Can you work these out from the model? Positions are in its coordinate system, mm. A direction names the side the tool comes from. Give positions to 0.01 mm unless a question says otherwise; leave off trailing zeros. Loops run counter-clockwise (first coordinate to the right, second up) from the corner with the lowest first, then second, coordinate; pieces in that order, holes last. Notation, with made-up numbers: M -12,43 L 8,43 A29 ccw 8,67 Z; hole C 85,-28 d10. An arc over 180 degrees is marked long. Put each result on its own line as item: value. Start each with the question number.
1) Imagine slicing it at D-D (z = 18). Write out the boundary of the cut face in (x, y), then the cut area to 3 significant figures.
2) If we mould it in two halves opening along Y, with no side actions, what happens to faces 1 (the flat face through (-24, -25, 12)), 2 (the flat face through (0, 3, 9)), 3 (the flat face through (0, 6, 0))? For each: +Y half, -Y half, draft (parallel to the pull), parting line (faces both ways), or undercut.
3) For P1, Ø10, axis at y = -48, z = -5, coming from the +X side; P2, Ø20, axis at x = 5, z = -0.5, coming from the -Y side; P3, Ø3, axis at x = 14.5, y = 4, coming from the +Z side; P4, Ø1.5, axis at x = -25.5, y = -4, coming from the -Z side, each with a flat end and sliding along its axis, tell me the tip position at first contact or that it passes through.
4) Imagine slicing it at C-C (x = 13). Write out the boundary of the cut face in (y, z).
5) For faces 4 (the flat face through (-27, -37, -4)), 5 (the cylindrical face through (-29.458, -20.062, 26.795)), 6 (the flat face through (-20.5, -40, 12)), which set-ups out of +Z, -Z, +X, -X, +Y, -Y let a thin tool reach every point of the face, with its end or its side?
6) Imagine slicing it at B-B (y = -32.5). Write out the boundary of the cut face in (x, z).
7) Please list where these lines run through material, in increasing order: line 1 along X through (y, z) = (-9, 2.5); line 2 along X through (y, z) = (-43.5, 20); line 3 along Y through (x, z) = (18, -6). Write a range as from..to.
8) Imagine slicing it at A-A (z = 6.5). Write out the boundary of the cut face in (x, y), then the cut area to 3 significant figures.
from build123d import *

# Parameters (mm, degrees)
SKETCH1_W           = 65
SKETCH1_H           = 18
BOSS_EXTRUDE1_DEPTH = 6
BOSS_EXTRUDE2_DEPTH = 6
FILLET1_R           = 10
FILLET3_R           = 3
SKETCH3_W           = 31
SKETCH3_H           = 31
BOSS_EXTRUDE3_DEPTH = 6


with BuildPart() as part:
    # Sketch1 → Boss-Extrude1 (new body)
    with BuildSketch(Plane(origin=(0, 0, 0), x_dir=(1, 0, 0), z_dir=(0, 1, 0))):
        Rectangle(SKETCH1_W, SKETCH1_H)
    extrude(amount=BOSS_EXTRUDE1_DEPTH)

    # Sketch2 → Boss-Extrude2 (add)
    with BuildSketch(Plane.ZY.offset(32.5)):
        Polygon((9, 0), (-9, 0), (-4, -5), (-4, -56), (27, -56), (27, -20), align=None)
    extrude(amount=-BOSS_EXTRUDE2_DEPTH)

    # Fillet1
    fillet1_edges = [part.edges().sort_by_distance(p)[0] for p in [
        (-29.5, 0, 9),
    ]]
    fillet(fillet1_edges, radius=FILLET1_R)

    # Fillet3
    fillet3_edges = [part.edges().sort_by_distance(p)[0] for p in [
        (-29.5, -20, 27),
        (-29.5, -5, -4),
    ]]
    fillet(fillet3_edges, radius=FILLET3_R)

    # Sketch3 → Boss-Extrude3 (add)
    with BuildSketch(Plane(origin=(-26.5, 0, 0), x_dir=(0, 0, -1), z_dir=(1, 0, 0))):
        with Locations((-11.5, -40.5)):
            Rectangle(SKETCH3_W, SKETCH3_H)
    extrude(amount=BOSS_EXTRUDE3_DEPTH)


solid = part.part
Recorded:
1. outline: M -32.5,-56 L -20.5,-56 L -20.5,-25 L -26.5,-25 L -26.5,-10 L -32.5,-10 Z
1. area: 462 mm²
2. face 1: undercut
2. face 2: draft
2. face 3: +Y half
3. P1: x = -20.5
3. P2: y = 0
3. P3: z = 9
3. P4: through
4. outline: M 0,-9 L 6,-9 L 6,9 L 0,9 Z
5. face 4: -Z, +X, -X, -Y
5. face 5: +Z, +X, -X, +Y
5. face 6: +Z, -Z, +X, -Y
6. outline: M -32.5,-4 L -20.5,-4 L -20.5,27 L -32.5,27 Z
7. line 1: -32.5..-26.5
7. line 2: -32.5..-20.5
7. line 3: 0..6
8. outline: M -32.5,-56 L -20.5,-56 L -20.5,-25 L -26.5,-25 L -26.5,0 L 32.5,0 L 32.5,6 L -32.5,6 Z
8. area: 912 mm²
